```python
from build123d import *

# Parameters (mm, degrees)
LINEAR_AUSTRAGEN_D_NN1_DEPTH = 2.5


with BuildPart() as part:
    # Skizze1 → Linear-Austragen-Dünn1 (new, symmetric)
    with BuildSketch(Plane.XY):
        with BuildLine():
            Line((233.5, 326.961421282), (233.5, 294.5770817))
            Line((233.5, 294.5770817), (247.5, 27.187011832))
            Line((247.5, 27.187011832), (247.5, 0))
            ThreePointArc((247.5, 0), (245.303300859, -5.303300859), (240, -7.5))
            Line((240, -7.5), (-240, -7.5))
            ThreePointArc((-240, -7.5), (-245.303300859, -5.303300859), (-247.5, 0))
            Line((-247.5, 0), (-247.5, 480))
            ThreePointArc((-247.5, 480), (-240, 487.5), (-232.5, 480))
            Line((-232.5, 480), (-232.5, 280))
            Line((-232.5, 280), (-232, 280))
            Line((-232, 280), (-232, 480))
            ThreePointArc((-232, 480), (-240, 488), (-248, 480))
            Line((-248, 480), (-248, 0))
            ThreePointArc((-248, 0), (-245.656854249, -5.656854249), (-240, -8))
            Line((-240, -8), (240, -8))
            ThreePointArc((240, -8), (245.656854249, -5.656854249), (248, 0))
            Line((248, 0), (248, 27.200092364))
            Line((248, 27.200092364), (234, 294.590162233))
            Line((234, 294.590162233), (234, 326.961421282))
            Line((234, 326.961421282), (233.5, 326.961421282))
        make_face()
    extrude(amount=LINEAR_AUSTRAGEN_D_NN1_DEPTH, both=True)


solid = part.part
```
Source: CAD feature listing. Evaluate the final solid. Frame: model axes, mm. Coordinates: 2 decimals unless noted, no trailing zeros. Order: outer loops, then holes, each group sorted by start corner. A loop starts at its lowest first (then second) coordinate and runs counter-clockwise, first axis right, second up. Notation, with made-up numbers: M -23,-1.5 L -5,-1.5 A30 ccw -5,34.5 Z; hole C 64,21.25 d7. An arc over 180 degrees is marked long. Write each question's results on one line, items separated by ' | '. Start each with the question number.
1) Draft query along X for faces 1 (the face through (241.1, 159, 0)), 2 (the face through (240.4, 162.8, 0)). Return one class per face: released by +X, released by -X, zero draft, split by the parting line, or undercut.
2) Section query B-B (x = 151). Return the cut outline in (y, z), plus the area to 3 significant figures.
3) Section query A-A (y = 49.5). Return the cut outline in (x, z).
4) Contact query for flat-ended pins moving along their axis: pin 1 Ø1.5 at (x, z) = (11, -1.5) entering from +Y; pin 2 Ø0.6 at (x, z) = (234, -1) entering from +Y; pin 3 Ø2.5 at (y, z) = (305.5, 0) entering from +X. Output: stop coordinate, or through.
5) Line query: line 1 (X direction, y = 313.5, z = -2.1); line 2 (X direction, y = 332.5, z = 1.7); line 3 (X direction, y = 234.5, z = -2.3). Output: solid intervals per line, ascending. Write a range as from..to.
Answers:
1) face 1: released by +X | face 2: undercut
2) outline: M -8,-2.5 L -7.5,-2.5 L -7.5,2.5 L -8,2.5 Z | area: 2.50 mm^2
3) outline: M -248,-2.5 L -247.5,-2.5 L -247.5,2.5 L -248,2.5 Z; M 246.33,-2.5 L 246.83,-2.5 L 246.83,2.5 L 246.33,2.5 Z
4) pin 1: stops at y = -7.5 | pin 2: stops at y = 326.96 | pin 3: stops at x = 234
5) line 1: x = -248..-247.5, -232.5..-232, 233.5..234 | line 2: x = -248..-247.5, -232.5..-232 | line 3: x = -248..-247.5, 236.65..237.15
